from build123d import *

# Parameters (mm, degrees)
SKETCH_1_R          = 25
SKETCH_1_R_2        = 2.05
EXTRUDE_1_DEPTH     = 6
SKETCH_2_R          = 15
CUT_EXTRUDE_1_DEPTH = 36.860842154


with BuildPart() as part:
    # 草图1 → 凸台-拉伸1 (new body)
    with BuildSketch(Plane(origin=(0, 0, 0), x_dir=(1, 0, 0), z_dir=(0, 1, 0))):
        with Locations(Location((0, 0, 0), (0, 0, 270))):
            Circle(SKETCH_1_R)
        with Locations(Location((-15, 15, 0), (0, 0, 270))):
            Circle(SKETCH_1_R_2, mode=Mode.SUBTRACT)
        with Locations(Location((15, 15, 0), (0, 0, 270))):
            Circle(SKETCH_1_R_2, mode=Mode.SUBTRACT)
        with Locations(Location((15, -15, 0), (0, 0, 270))):
            Circle(SKETCH_1_R_2, mode=Mode.SUBTRACT)
        with Locations(Location((-15, -15, 0), (0, 0, 270))):
            Circle(SKETCH_1_R_2, mode=Mode.SUBTRACT)
    extrude(amount=EXTRUDE_1_DEPTH)

    # 草图2 → 切除-拉伸1 (cut, through all)
    with BuildSketch(Plane(origin=(0, 6, 0), x_dir=(1, 0, 0), z_dir=(0, 1, 0))):
        with Locations(Location((0, 0, 0), (0, 0, 270))):
            Circle(SKETCH_2_R)
    extrude(amount=-CUT_EXTRUDE_1_DEPTH, mode=Mode.SUBTRACT)


solid = part.part
CAD build for the part. Positions are in the model's coordinates, mm. Give positions to 0.01 mm unless a question says otherwise; leave off trailing zeros. Write each loop counter-clockwise with the first axis right and the second up, starting at its lowest first coordinate (ties: lowest second). Pieces come first, ordered by that corner, then holes. Notation, with made-up numbers: (86.5, -11) - (133.5, -11) arc R17 cw to (133.5, 2) - close; hole circle Ø1 at (84, 35). An arc over 180 degrees is marked (long way). Put each result on its own line as item: value.
(1) Drop flat-ended pins along their axis: pin 1 Ø1.5 at (x, y) = (19.5, 4.5) entering from +Z; pin 2 Ø1 at (y, z) = (2, -2.5) entering from +X; pin 3 Ø2 at (x, y) = (-10, 3) entering from +Z. Give the stop position or say it passes through.
Working result:
pin 1: z = 16.54
pin 2: x = 24.92
pin 3: z = 23.32
(2) Saw through at D-D (x = -16). List the corners of the cut face in (y, z), then the cut area to 3 significant figures.
Working result:
outline: (0, -19.21) - (6, -19.21) - (6, -16.79) - (0, -16.79) - close; (0, -13.21) - (6, -13.21) - (6, 13.21) - (0, 13.21) - close; (0, 16.79) - (6, 16.79) - (6, 19.21) - (0, 19.21) - close
area: 188 mm^2
(3) Pull direction X, two halves, no side cores. Call faces 1 (the flat face through (-11, 6, 11)), 2 (the cylindrical face through (7.509, 2.958, 23.846)), 3 (the cylindrical face through (15.09, 2.96, 12.95)): released by +X, released by -X, zero draft, split by the parting line, or undercut.
Working result:
face 1: zero draft
face 2: split by the parting line
face 3: undercut
(4) Saw through at A-A (z = 0). List the corners of the cut face in (x, y), then the cut area to 3 significant figures.
Working result:
outline: (-25, 0) - (-15, 0) - (-15, 6) - (-25, 6) - close; (15, 0) - (25, 0) - (25, 6) - (15, 6) - close
area: 120 mm^2
(5) Wall check: L1, parallel to X at y = 0.35, z = 16; L2, parallel to X at y = 3.85, z = 0; L3, parallel to X at y = 4.4, z = -16.5. Give the ranges that are in metal, low to high.
Working result:
L1: -19.21 to -16.79, -13.21 to 13.21, 16.79 to 19.21
L2: -25 to -15, 15 to 25
L3: -18.78 to -16.4, -13.6 to 13.6, 16.4 to 18.78
(6) Saw through at B-B (x = 0). List the corners of the cut face in (y, z), then the cut area to 3 significant figures.
Working result:
outline: (0, -25) - (6, -25) - (6, -15) - (0, -15) - close; (0, 15) - (6, 15) - (6, 25) - (0, 25) - close
area: 120 mm^2
(7) Saw through at C-C (y = 3.45). List the corners of the cut face in (x, z), then the cut area to 3 significant figures.
Working result:
outline: circle Ø50 at (0, 0); hole circle Ø4.1 at (-15, -15); hole circle Ø4.1 at (-15, 15); hole circle Ø30 at (0, 0); hole circle Ø4.1 at (15, -15); hole circle Ø4.1 at (15, 15)
area: 1,200 mm^2
